Source: CAD feature listing. Evaluate the final solid. Frame: model axes, mm. A direction names the side the tool comes from. Give positions to 0.01 mm unless a question says otherwise; leave off trailing zeros. Order: outer loops, then holes, each group sorted by start corner. A loop starts at its lowest first (then second) coordinate and runs counter-clockwise, first axis right, second up.
from build123d import *

# Parameters (mm, degrees)
BOSS_EXTRUDE1_DEPTH = 10
FILLET1_R           = 6
FILLET2_R           = 2
FILLET3_R           = 2


with BuildPart() as part:
    # Sketch1 → Boss-Extrude1 (new body)
    with BuildSketch(Plane.XY):
        with BuildLine():
            Line((-27.171188048, -9.347902097), (-27.171188048, -6.180932375))
            ThreePointArc((-27.171188048, -6.180932375), (-27.771188048, -4.347902097), (-27.171188048, -2.514871819))
            Line((-27.171188048, -2.514871819), (-27.171188048, 4.485128181))
            Line((-27.171188048, 4.485128181), (-22.171188048, 4.485128181))
            Line((-22.171188048, 4.485128181), (-22.171188048, -2.514871819))
            ThreePointArc((-22.171188048, -2.514871819), (-21.725004076, -3.38353702), (-21.571188048, -4.347902097))
            ThreePointArc((-21.571188048, -4.347902097), (-21.725004076, -5.312267173), (-22.171188048, -6.180932375))
            Line((-22.171188048, -6.180932375), (-22.171188048, -9.347902097))
            Line((-22.171188048, -9.347902097), (-19.171188048, -9.347902097))
            Line((-19.171188048, -9.347902097), (-19.171188048, 7.485128181))
            Line((-19.171188048, 7.485128181), (-30.171188048, 7.485128181))
            Line((-30.171188048, 7.485128181), (-30.171188048, -9.347902097))
            Line((-30.171188048, -9.347902097), (-27.171188048, -9.347902097))
        make_face()
    extrude(amount=BOSS_EXTRUDE1_DEPTH)

    # Fillet1
    # the kernel refuses this fillet: 6 mm, written as the material it takes off along each edge
    with BuildSketch(Plane(origin=(-19.171188048, 7.485128181, -15), x_dir=(-1, 0, 0), z_dir=(0, 0, 1))) as fillet1_piece_1:
        with BuildLine():
            CenterArc((FILLET1_R, FILLET1_R), FILLET1_R, 180, 90)
            Line((0, FILLET1_R), (0, 0))
            Line((0, 0), (FILLET1_R, 0))
        make_face()
    extrude(amount=40, mode=Mode.SUBTRACT)
    with BuildSketch(Plane(origin=(-30.171188048, 7.485128181, -15), x_dir=(1, 0, 0), z_dir=(0, 0, 1))) as fillet1_piece_2:
        with BuildLine():
            CenterArc((FILLET1_R, -FILLET1_R), FILLET1_R, 90, 90)
            Line((0, -FILLET1_R), (0, 0))
            Line((0, 0), (FILLET1_R, 0))
        make_face()
    extrude(amount=40, mode=Mode.SUBTRACT)

    # Fillet2
    # the kernel refuses this fillet: 2 mm, written as the material it takes off along each edge
    with BuildSketch(Plane(origin=(-19.171188048, -9.347902097, -5), x_dir=(0, 1, 0), z_dir=(0, 0, 1)), Plane(origin=(-22.171188048, -9.347902097, -5), x_dir=(1, 0, 0), z_dir=(0, 0, 1)), Plane(origin=(-30.171188048, -9.347902097, -5), x_dir=(1, 0, 0), z_dir=(0, 0, 1))) as fillet2_piece_1:
        with BuildLine():
            CenterArc((FILLET2_R, FILLET2_R), FILLET2_R, 180, 90)
            Line((0, FILLET2_R), (0, 0))
            Line((0, 0), (FILLET2_R, 0))
        make_face()
    extrude(amount=20, mode=Mode.SUBTRACT)
    with BuildSketch(Plane(origin=(-27.171188048, -9.347902097, -5), x_dir=(-1, 0, 0), z_dir=(0, 0, 1))) as fillet2_piece_2:
        with BuildLine():
            CenterArc((FILLET2_R, -FILLET2_R), FILLET2_R, 90, 90)
            Line((0, -FILLET2_R), (0, 0))
            Line((0, 0), (FILLET2_R, 0))
        make_face()
    extrude(amount=20, mode=Mode.SUBTRACT)

    # Fillet3
    fillet3_edges = [part.edges().sort_by_distance(p)[0] for p in [
        (-22.171188048, 4.485128181, 5),
        (-27.171188048, 4.485128181, 5),
    ]]
    fillet(fillet3_edges, radius=FILLET3_R)


solid = part.part
1) First-contact query: pin 1 Ø0.8 at (x, z) = (-24.5, 3.5) entering from -Y. Flat tip, straight axial feed; report the tip coordinate or a pass-through.
Checks:
pin 1: stops at y = 4.48
2) Ray query, L1, parallel to X at y = -4.5, z = 8.5; L2, parallel to X at y = -1.5, z = 6.75; L3, parallel to X at y = 5, z = 5. Return the intervals inside material, ascending.
Checks:
L1: x = -30.17 to -27.77, -21.57 to -19.17
L2: x = -30.17 to -27.17, -22.17 to -19.17
L3: x = -29.03 to -20.31
3) Section query D-D on x = -26. Output: boundary loops of the cut face in (y, z), and give its area (3 significant figures).
Checks:
outline: (4.31, 0) - (7.2, 0) - (7.2, 10) - (4.31, 10) - close
area: 28.9 mm2
4) Section query B-B on z = 7.5. Output: boundary loops of the cut face in (x, y), and give its area (3 significant figures).
Checks:
outline: (-30.17, -7.35) arc R2 ccw to (-28.67, -9.28) arc R2 ccw to (-27.17, -7.35) - (-27.17, -6.18) arc R3.1 cw to (-27.17, -2.51) - (-27.17, 2.49) arc R2 cw to (-25.17, 4.49) - (-24.17, 4.49) arc R2 cw to (-22.17, 2.49) - (-22.17, -2.51) arc R3.1 cw to (-22.17, -6.18) - (-22.17, -7.35) arc R2 ccw to (-20.67, -9.28) arc R2 ccw to (-19.17, -7.35) - (-19.17, 1.49) arc R6 ccw to (-24.67, 7.46) arc R6 ccw to (-30.17, 1.49) - close
area: 95.9 mm2
5) Reachability of faces 1 (the face through (-19.601, -8.587, 4.93)), 2 (the face through (-22.74, 3.88, 5.07)) from +Z, -Z, +X, -X, +Y, -Y: full face, straight path, thin tool, end or side. Return the list, or none.
Checks:
face 1: +Z, -Z, +X, -Y
face 2: +Z, -Z, -Y
6) Pull-direction query (Y, two-part tool) for faces 3 (the face through (-21.76, -8.56, 4.93)), 4 (the face through (-28.545, 5.593, 4.93)), 5 (the face through (-27.77, -4.38, 4.93)), 6 (the face through (-22.171, 0, 5)); classes: +Y half, -Y half, draft (parallel to the pull), parting line (faces both ways), or undercut.
Checks:
face 3: -Y half
face 4: +Y half
face 5: undercut
face 6: draft
7) Section query C-C on x = -27.5. Output: boundary loops of the cut face in (y, z).
Checks:
outline: (-8.45, 0) - (-5.62, 0) - (-5.62, 10) - (-8.45, 10) - close; (-3.08, 0) - (6.48, 0) - (6.48, 10) - (-3.08, 10) - close
8) Section query A-A on y = -0.25. Output: boundary loops of the cut face in (x, z).
Checks:
outline: (-30.17, 0) - (-27.17, 0) - (-27.17, 10) - (-30.17, 10) - close; (-22.17, 0) - (-19.17, 0) - (-19.17, 10) - (-22.17, 10) - close
